from build123d import *

# Parameters (mm, degrees)
F0_R     = 9
F1_DEPTH = 28
F0_R_2   = 5
F0_R_3   = 6
F2_DEPTH = 10


with BuildPart() as f1:
    # F0 (on Top) → F1 (new body)
    with BuildSketch(Plane.XY):
        with BuildLine():
            ThreePointArc((-0.923077, 14.971571), (-10.275063, -10.928087), (15, 0))
            ThreePointArc((15, 0), (14.773901, 2.594582), (14.102419, 5.110947))
            ThreePointArc((14.102419, 5.110947), (8.22993, 12.540664), (-0.923077, 14.971571))
        make_face()
        Circle(F0_R, mode=Mode.SUBTRACT)
    extrude(amount=F1_DEPTH)

    # F0 (on Top) → F2 (join)
    with BuildSketch(Plane.XY):
        with BuildLine():
            ThreePointArc((-0.923077, 14.971571), (-10.275063, -10.928087), (15, 0))
            ThreePointArc((15, 0), (14.773901, 2.594582), (14.102419, 5.110947))
            ThreePointArc((14.102419, 5.110947), (8.22993, 12.540664), (-0.923077, 14.971571))
        make_face()
        Circle(F0_R, mode=Mode.SUBTRACT)
        with BuildLine():
            ThreePointArc((14.102419, 5.110947), (14.773901, 2.594582), (15, 0))
            ThreePointArc((15, 0), (-10.275063, -10.928087), (-0.923077, 14.971571))
            Line((-0.923077, 14.971571), (-65.676923, 10.979152))
            ThreePointArc((-65.676923, 10.979152), (-76, 0), (-65.676923, -10.979152))
            Line((-65.676923, -10.979152), (-11.616035, -14.312293))
            ThreePointArc((-11.616035, -14.312293), (-7.734373, -15.361567), (-4.579807, -17.854954))
            Line((-4.579807, -17.854954), (13.87871, -39.791725))
            ThreePointArc((13.87871, -39.791725), (24, -41.569219), (27.52129, -31.915178))
            Line((27.52129, -31.915178), (14.102419, 5.110947))
        make_face()
        with Locations((20, -34.641016)):
            Circle(F0_R_2, mode=Mode.SUBTRACT)
        with Locations((-65, 0)):
            Circle(F0_R_3, mode=Mode.SUBTRACT)
    extrude(amount=F2_DEPTH)


solid = f1.part
Part model, mm, in its own coordinate system. A direction names the side the tool comes from. Coordinates: 2 decimals unless noted, no trailing zeros. Write each loop counter-clockwise with the first axis right and the second up, starting at its lowest first coordinate (ties: lowest second). Pieces come first, ordered by that corner, then holes. Notation, with made-up numbers: (46, 85) - (80, 85) arc R28 ccw to (80, 121) - close; hole circle Ø11 at (23, -21.5). An arc over 180 degrees is marked (long way). Put each result on its own line as item: value.
1. Band-saw the part on B-B (y = -36). Write the cut outline in (x, z).
Final values:
outline: (10.69, 0) - (15.19, 0) - (15.19, 10) - (10.69, 10) - close; (24.81, 0) - (27.88, 0) - (27.88, 10) - (24.81, 10) - close
2. Probe line 1 along Y through (x, z) = (0, 13.5); line 2 along Z through (x, y) = (-51.5, -8); line 3 along X through (y, z) = (-7, 24.75). List the from-to ranges inside material, lowest first. Write a range as [from, to].
Final values:
line 1: y = [-15, -9], [9, 15]
line 2: z = [0, 10]
line 3: x = [-13.27, -5.66], [5.66, 13.27]
3. Two-plate mould, pull along Y, no slides. Class faces 1 (the cylindrical face through (-1.172, 8.923, 13.804)), 2 (the cylindrical face through (-71, 0, 5)), 3 (the cylindrical face through (-76, 0, 5)), 4 (the flat face through (-24, -9, 10)): +Y half, -Y half, draft (parallel to the pull), parting line (faces both ways), or undercut.
Final values:
face 1: undercut
face 2: undercut
face 3: parting line
face 4: draft
4. Band-saw the part on A-A (x = 20.5). Write the cut outline in (y, z), then the cut area to 3 significant figures.
Final values:
outline: (-42.63, 0) - (-39.62, 0) - (-39.62, 10) - (-42.63, 10) - close; (-29.67, 0) - (-12.54, 0) - (-12.54, 10) - (-29.67, 10) - close
area: 201 mm²
5. Flat gauge pins, fed straight in: pin 1 Ø6 at (x, y) = (2, -22.5) entering from +Z; pin 2 Ø10 at (x, z) = (-44, 12.5) entering from -Y; pin 3 Ø3 at (x, z) = (-5.5, 24.5) entering from -Y; pin 4 Ø20.5 at (x, y) = (0, 0) entering from -Z. Where does each tip first touch, or does it go through?
Final values:
pin 1: stops at z = 10
pin 2: stops at y = -12.58
pin 3: stops at y = -14.46
pin 4: stops at z = 0
6. Band-saw the part on D-D (z = 7.25). Write the cut outline in (x, y).
Final values:
outline: (-65.68, -10.98) - (-11.62, -14.31) arc R10 cw to (-4.58, -17.85) - (13.88, -39.79) arc R8 ccw to (27.52, -31.92) - (14.1, 5.11) arc R15 ccw to (-0.92, 14.97) - (-65.68, 10.98) arc R11 ccw to start; hole circle Ø12 at (-65, 0); hole circle Ø18 at (0, 0); hole circle Ø10 at (20, -34.64)
7. 3-axis set-ups, long thin cutter, end or side, ignore diameter. For faces 5 (the cylindrical face through (14.78, 2.56, 18.87)), 6 (the flat face through (6.5, -6.5, 28)): which of +Z, -Z, +X, -X, +Y, -Y reach the whole face in a straight line?
Final values:
face 5: +Z, +X, +Y
face 6: +Z, +X, -X, +Y, -Y
8. Band-saw the part on C-C (z = 25.5). Write the cut outline in (x, y), then the cut area to 3 significant figures.
Final values:
outline: (14.1, 5.11) arc R15 ccw (long way) to (15, 0) arc R15 ccw to start; hole circle Ø18 at (0, 0)
area: 452 mm²
